Source: CAD feature listing. Evaluate the final solid. Frame: model axes, mm. Face numbers are marked on the shaded views. A direction names the side the tool comes from. Coordinates: 2 decimals unless noted, no trailing zeros. Write each loop counter-clockwise with the first axis right and the second up, starting at its lowest first coordinate (ties: lowest second). Pieces come first, ordered by that corner, then holes. Notation, with made-up numbers: M -29.75,21 L 10.25,21 A13 cw 10.25,41 Z; hole C -4,69 d5. An arc over 180 degrees is marked long. Answer as CSV lines item,"result". Start each with the question number.
1. Reachability of the marked faces 4, 5 and 6 from +Z, -Z, +X, -X, +Y, -Y: full face, straight path, thin tool, end or side. Return the list, or none.
2. Section C-C on z = -5. Return the cut outline in (x, y) (3 decimals).
3. Line query: probe 1 along Y at (x, z) = (21, 0); probe 2 along X at (y, z) = (28, 2) (3 decimals); probe 3 along X at (y, z) = (15, -12). Output: solid intervals per line, ascending. Write a range as [from, to].
4. Section D-D on z = 10. Return the cut outline in (x, y), plus the area to 3 significant figures.
5. Contact query for flat-ended pins moving along their axis: pin 1 Ø1 at (y, z) = (30, 13.5) entering from +X; pin 2 Ø5 at (x, y) = (-7.5, 34) entering from +Z; pin 3 Ø16 at (x, y) = (-19.83, 19.05) entering from -Z; pin 4 Ø17 at (x, z) = (0, 0) entering from +Y. Output: stop coordinate, or through.
6. Section B-B on y = 33.5. Return the cut outline in (x, z) (1 decimal), plus the area to 3 significant figures.
7. Mould query, pull axis Z, two halves, no side actions, for the marked faces 1, 2 and 3. Classes: pulls with the +Z half, pulls with the -Z half, needs draft (parallel to the pull), parting line crosses it, or undercut.
8. Section A-A on x = 8.5. Return the cut outline in (y, z).
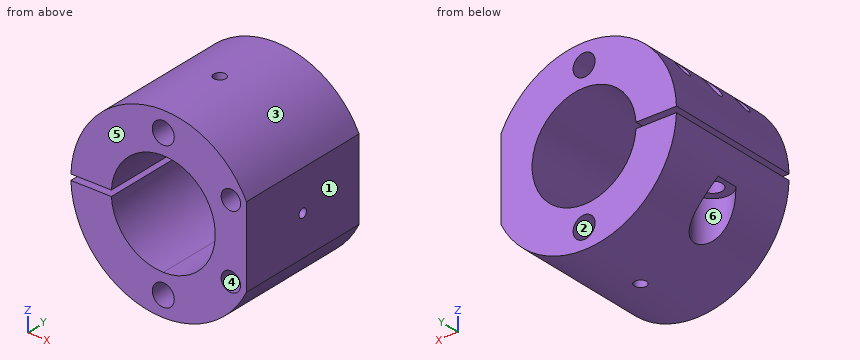
```python
from build123d import *

# Parameters (mm, degrees)
SKETCH2_R                        = 25.4
SKETCH2_R_2                      = 14.2875
BOSS_EXTRUDE1_DEPTH              = 38.1
CUT_EXTRUDE1_REACH               = 54.363
SKETCH3_W                        = 25.4
SKETCH3_H                        = 1.5875
CUT_EXTRUDE2_REACH               = 54.363
SKETCH4_R                        = 3.0226
TAP_DRILL_FOR_M4X0_7_TAP1_REACH  = 61.824
TAP_DRILL_FOR_M4X0_7_TAP1_BORE_R = 1.65
CUT_EXTRUDE5_REACH               = 70.392
CUT_EXTRUDE5_END_RADIUS          = 3.0226
SKETCH11_R                       = 1.65
CUT_EXTRUDE6_REACH               = 54.363
TAP_DRILL_FOR_M3X0_5_TAP2_D      = 2.5
TAP_DRILL_FOR_M3X0_5_TAP2_DEPTH  = 4.572
TAP_DRILL_FOR_M3X0_5_TAP2_TIP    = 0.751075774
TAP_DRILL_FOR_M5X0_8_TAP1_REACH  = 55.583
TAP_DRILL_FOR_M5X0_8_TAP1_BORE_R = 2.1
SKETCH15_R                       = 2.665
CUT_EXTRUDE7_DEPTH               = 53.7470617
CUT_EXTRUDE8_REACH               = 59.143
SKETCH19_R                       = 5
SKETCH21_R                       = 2.665
CUT_EXTRUDE10_DEPTH              = 10


with BuildPart() as part:
    # Sketch2 → Boss-Extrude1 (new body)
    with BuildSketch(Plane(origin=(0, 0, 0), x_dir=(1, 0, 0), z_dir=(0, 1, 0))):
        with Locations(Location((0, 0, 0), (0, 0, 90))):
            Circle(SKETCH2_R)
        with Locations(Location((0, 0, 0), (0, 0, 90))):
            Circle(SKETCH2_R_2, mode=Mode.SUBTRACT)
    extrude(amount=BOSS_EXTRUDE1_DEPTH)

    # Sketch3 → Cut-Extrude1 (cut, up to next)
    with BuildSketch(Plane(origin=(0, 38.1, 0), x_dir=(1, 0, 0), z_dir=(0, 1, 0)), mode=Mode.PRIVATE) as cut_extrude1_sk1:
        with Locations((-12.7, 0)):
            Rectangle(SKETCH3_W, SKETCH3_H)
    cut_extrude1_tool1 = extrude(cut_extrude1_sk1.sketch, amount=-CUT_EXTRUDE1_REACH, mode=Mode.PRIVATE) & part.part
    add(cut_extrude1_tool1.solids().sort_by_distance((-12.7, 38.1, 0))[0], mode=Mode.SUBTRACT)

    # Sketch4 → Cut-Extrude2 (cut, up to next)
    with BuildSketch(Plane(origin=(0, 38.1, 0), x_dir=(1, 0, 0), z_dir=(0, 1, 0)), mode=Mode.PRIVATE) as cut_extrude2_sk1:
        with Locations(Location((0, -19.84375, 0), (0, 0, 270))):
            Circle(SKETCH4_R)
    cut_extrude2_tool1 = extrude(cut_extrude2_sk1.sketch, amount=-CUT_EXTRUDE2_REACH, mode=Mode.PRIVATE) & part.part
    cut_extrude2 = cut_extrude2_tool1.solids().sort_by_distance((0, 38.1, 19.84375))[0]
    add(cut_extrude2, mode=Mode.SUBTRACT)

    # Tap Drill for M4x0.7 Tap1 bore (on position points) → Tap Drill for M4x0.7 Tap1 (cut, up to next)
    with BuildSketch(Plane(origin=(-19.826514488, 29.109235595, 0.79375), x_dir=(-1, 0, 0), z_dir=(0, 0, -1)), mode=Mode.PRIVATE) as tap_drill_for_m4x0_7_tap1_sk1:
        Circle(TAP_DRILL_FOR_M4X0_7_TAP1_BORE_R)
    tap_drill_for_m4x0_7_tap1_tool1 = extrude(tap_drill_for_m4x0_7_tap1_sk1.sketch, amount=-TAP_DRILL_FOR_M4X0_7_TAP1_REACH, mode=Mode.PRIVATE) & part.part
    # Tap Drill for M4x0.7 Tap1 bore (on position points) → Tap Drill for M4x0.7 Tap1 (cut, up to next)
    with BuildSketch(Plane(origin=(-19.826514488, 29.109235595, 0.79375), x_dir=(-1, 0, 0), z_dir=(0, 0, -1)), mode=Mode.PRIVATE) as tap_drill_for_m4x0_7_tap1_sk2:
        with Locations((0, -20.205281104)):
            Circle(TAP_DRILL_FOR_M4X0_7_TAP1_BORE_R)
    tap_drill_for_m4x0_7_tap1_tool2 = extrude(tap_drill_for_m4x0_7_tap1_sk2.sketch, amount=-TAP_DRILL_FOR_M4X0_7_TAP1_REACH, mode=Mode.PRIVATE) & part.part
    add(tap_drill_for_m4x0_7_tap1_tool1.solids().sort_by_distance((-19.826514, 29.109236, 0.79375))[0], mode=Mode.SUBTRACT)
    add(tap_drill_for_m4x0_7_tap1_tool2.solids().sort_by_distance((-19.826514, 8.903954, 0.79375))[0], mode=Mode.SUBTRACT)

    # Cut-Extrude5: up to this cylinder (the profile starts outside it)
    cut_extrude5_end = Plane(origin=(0, 19.05, 19.84375), z_dir=(0, 1, 0)) * Cylinder(CUT_EXTRUDE5_END_RADIUS, 147.8292, mode=Mode.PRIVATE)
    # Sketch11 → Cut-Extrude5 (cut, up to the surface)
    with BuildSketch(Plane.XY.offset(25.4), mode=Mode.PRIVATE) as cut_extrude5_sk1:
        with Locations((0.006202687, 19.05)):
            Circle(SKETCH11_R)
    cut_extrude5_tool1 = extrude(cut_extrude5_sk1.sketch, amount=-CUT_EXTRUDE5_REACH, mode=Mode.PRIVATE) - cut_extrude5_end
    cut_extrude5 = cut_extrude5_tool1.solids().sort_by_distance((0.006203, 19.05, 25.4))[0]
    add(cut_extrude5, mode=Mode.SUBTRACT)

    # Mirror1: Cut-Extrude2, Cut-Extrude5 across plane
    add(cut_extrude2.mirror(Plane.XY), mode=Mode.SUBTRACT)
    add(cut_extrude5.mirror(Plane.XY), mode=Mode.SUBTRACT)

    # Sketch12 → Cut-Extrude6 (cut, up to next)
    with BuildSketch(Plane(origin=(0, 38.1, 0), x_dir=(1, 0, 0), z_dir=(0, 1, 0)), mode=Mode.PRIVATE) as cut_extrude6_sk1:
        with BuildLine():
            Line((22.86, 11.071603317), (22.86, -11.071603317))
            ThreePointArc((22.86, -11.071603317), (25.4, 0), (22.86, 11.071603317))
        make_face()
    cut_extrude6_tool1 = extrude(cut_extrude6_sk1.sketch, amount=-CUT_EXTRUDE6_REACH, mode=Mode.PRIVATE) & part.part
    add(cut_extrude6_tool1.solids().sort_by_distance((23.880484, 38.1, 0))[0], mode=Mode.SUBTRACT)

    # Tap Drill for M3x0.5 Tap2
    with Locations(Plane(origin=(22.86, 19.05, 0), x_dir=(0, 0, 1), z_dir=(1, 0, 0))):
        with Locations((0, 0)):
            Hole(TAP_DRILL_FOR_M3X0_5_TAP2_D / 2, depth=TAP_DRILL_FOR_M3X0_5_TAP2_DEPTH)
            with Locations((0, 0, -(TAP_DRILL_FOR_M3X0_5_TAP2_DEPTH + TAP_DRILL_FOR_M3X0_5_TAP2_TIP / 2))):  # 118° drill point
                Cone(0, TAP_DRILL_FOR_M3X0_5_TAP2_D / 2, TAP_DRILL_FOR_M3X0_5_TAP2_TIP, mode=Mode.SUBTRACT)

    # Tap Drill for M5x0.8 Tap1 bore (on position points) → Tap Drill for M5x0.8 Tap1 (cut, up to next)
    with BuildSketch(Plane(origin=(-19.826514488, 19.05, 0.79375), x_dir=(-1, 0, 0), z_dir=(0, 0, -1)), mode=Mode.PRIVATE) as tap_drill_for_m5x0_8_tap1_sk1:
        Circle(TAP_DRILL_FOR_M5X0_8_TAP1_BORE_R)
    tap_drill_for_m5x0_8_tap1_tool1 = extrude(tap_drill_for_m5x0_8_tap1_sk1.sketch, amount=-TAP_DRILL_FOR_M5X0_8_TAP1_REACH, mode=Mode.PRIVATE) & part.part
    add(tap_drill_for_m5x0_8_tap1_tool1.solids().sort_by_distance((-19.826514, 19.05, 0.79375))[0], mode=Mode.SUBTRACT)

    # Sketch15 → Cut-Extrude7 (cut, through all)
    with BuildSketch(Plane(origin=(0, 0, 0.79375), x_dir=(-1, 0, 0), z_dir=(0, 0, -1))):
        with Locations(Location((19.826514488, 19.05, 0), (0, 0, 180))):
            Circle(SKETCH15_R)
    extrude(amount=CUT_EXTRUDE7_DEPTH, mode=Mode.SUBTRACT)

    # Sketch19 → Cut-Extrude8 (cut, up to next)
    with BuildSketch(Plane.XY.offset(-8.79375), mode=Mode.PRIVATE) as cut_extrude8_sk1:
        with Locations((-19.826514488, 19.05)):
            Circle(SKETCH19_R)
    cut_extrude8_tool1 = extrude(cut_extrude8_sk1.sketch, amount=-CUT_EXTRUDE8_REACH, mode=Mode.PRIVATE) & part.part
    add(cut_extrude8_tool1.solids().sort_by_distance((-19.826514, 19.05, -8.79375))[0], mode=Mode.SUBTRACT)

    # Sketch21 → Cut-Extrude10 (cut)
    with BuildSketch(Plane.XZ):
        with Locations(Location((18.57375, -10, 0), (0, 0, 270))):
            Circle(SKETCH21_R)
        with Locations(Location((18.57375, 10, 0), (0, 0, 90))):
            Circle(SKETCH21_R)
    extrude(amount=-CUT_EXTRUDE10_DEPTH, mode=Mode.SUBTRACT)


solid = part.part
```
Values:
1,face 4,"-Y"
1,face 5,"+Z, -Z, +X, -X, -Y"
1,face 6,"-Z"
2,outline,"M -24.903,0 L -13.384,0 L -13.384,38.1 L -24.903,38.1 Z; M 13.384,0 L 22.86,0 L 22.86,38.1 L 13.384,38.1 Z; hole C -19.827,19.05 d5.33"
3,probe 1,"[0, 17.8], [20.3, 38.1]"
3,probe 2,"[-25.321, -21.048], [-18.605, -14.147], [14.147, 22.86]"
3,probe 3,"[-16.89, -7.75], [7.75, 22.39]"
4,outline,"M -23.35,0 L -10.2,0 L -10.2,38.1 L -23.35,38.1 Z; M 10.2,0 L 15.91,0 L 15.91,10 L 21.24,10 L 21.24,0 L 22.86,0 L 22.86,38.1 L 10.2,38.1 Z; hole C -19.83,19.05 d4.2; hole C -19.83,8.9 d3.3; hole C -19.83,29.11 d3.3"
4,area,"899 mm²"
5,pin 1,"x = 21.82"
5,pin 2,"z = 24.9"
5,pin 3,"z = -22.48"
5,pin 4,"through"
6,outline,"M -25.4,-0.8 A25.4 ccw 22.9,-11.1 L 22.9,11.1 A25.4 ccw -25.4,0.8 L -14.3,0.8 A14.3 cw long -14.3,-0.8 Z; hole C 0,-19.8 d6; hole C 0,19.8 d6"
6,area,"1,270 mm²"
7,face 1,"needs draft"
7,face 2,"undercut"
7,face 3,"pulls with the +Z half"
8,outline,"M 0,-23.94 L 38.1,-23.94 L 38.1,-11.48 L 0,-11.48 Z; M 0,11.48 L 38.1,11.48 L 38.1,23.94 L 0,23.94 Z"
